Could you check a few things on this model? Use its own coordinates, in mm. Coordinates: 2 decimals unless noted, no trailing zeros. Order: outer loops, then holes, each group sorted by start corner. A loop starts at its lowest first (then second) coordinate and runs counter-clockwise, first axis right, second up. Notation, with made-up numbers: (75, 23.5) -> (115, 23.5) arc R13 ccw to (115, 32.5) -> close; hole circle Ø5 at (39.25, -37). An arc over 180 degrees is marked (long way). Use a Markdown table: item, result. Add a question column.
1) If I drill on L1, parallel to Y at x = 0, z = 1.7; L2, parallel to X at y = -20, z = 1.3; L3, parallel to X at y = -17.5, z = 1.8, over which ranges is the centre line in solid material (lowest first)? Write a range as [from, to].
2) Will this pin go through, and if not, where does the flat tip stop? pin 1 Ø6 at (x, y) = (0, -20) entering from -Z.
3) If we section it at A-A (x = -7): Write out the boundary of the cut face in (y, z).
Autodesk Inventor part; units mm, degrees
ref_plane "YZ Plane" through (0, 0, 0) normal (1, 0, 0) x (0, 1, 0)
ref_plane "XZ Plane" through (0, 0, 0) normal (0, 1, 0) x (-1, 0, 0)
ref_plane "XY Plane" through (0, 0, 0) normal (0, 0, 1) x (1, 0, 0)
sketch "Sketch1" plane through (0, 0, 0) normal (0, 0, 1) x (1, 0, 0)
  ellipse E0 centre (0, 0) end of major axis (90, 0) minor radius 60 (0, -60) -> (90, 0) ccw
  line L0 (0, 0) -> (90, 0)
  line L1 (0, -60) -> (0, 0)
  arc A0 (-34.5293, -41.1535) -> (0, -60) centre (0, -18.9457) ccw
  arc A1 (-30.6814, -11.8648) -> (-34.5293, -41.1535) centre (-15.2956, -28.7832) ccw
  arc A2 (0, 0) -> (-30.6814, -11.8648) centre (0, -45.6024) ccw
  point P0 (-30.1245, -11.3745)
  dimension "d0" = 90
  dimension "d1" = 60
extrude "Extrusion1" add sketch "Sketch1" along normal blind 3
fillet "Fillet1" radius 5 1 edges at (90, 0, 1.5)
sketch "Sketch2" plane through (0, 0, 3) normal (0, 0, 1) x (1, 0, 0)
  arc A0 (-1.5, -18) -> (1.5, -18) centre (0, -20) ccw
  line L0 (-1.5, -18) -> (1.5, -18)
  point P0 (0, 0)
  dimension "d5" = 5
  dimension "d6" = 20
  dimension "d7" = 2
extrude "Extrusion2" cut sketch "Sketch2" against normal blind 3
properties part number "cam3"
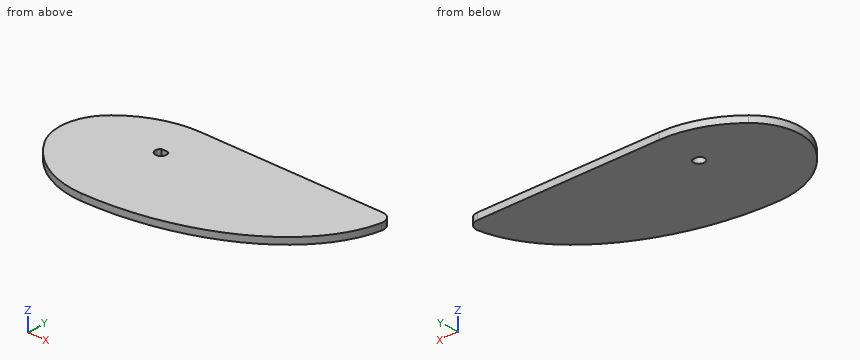
Answer sheet:
| question | item | result |
|---|---|---|
| 1 | L1 | [-60, -22.5], [-18, 0] |
| 1 | L2 | [-36.41, -2.5], [2.5, 84.85] |
| 1 | L3 | [-35.19, 86.09] |
| 2 | pin 1 | z = 0 |
| 3 | outline | (-59.4, 0) -> (-0.54, 0) -> (-0.54, 3) -> (-59.4, 3) -> close |
